Input: dimensioned drawing with shaded views. Units: mm. Origin: part minimum x, y, z. A direction names the side the tool comes from. Give positions to 0.01 mm unless a question says otherwise; leave off trailing zeros. Loops run counter-clockwise (first coordinate to the right, second up) from the corner with the lowest first, then second, coordinate; pieces in that order, holes last. Notation, with made-up numbers: (-32.75, -21) -> (-26.75, -21) arc R24 cw to (-26.75, 2) -> close; hole circle Ø1 at (-14, 72.25). An arc over 180 degrees is marked (long way). One line per question, with ' | ' between items. Start each with the question number.
Item 1: Section A-A on z = 254. Return loops of the section in (x, y) (3 decimals).
Item 2: Section D-D on z = 90. Return loops of the section in (x, y).
Item 3: Set-up query: the marked faces 1, 2, 3, 4 and 5. Return all of +Z, -Z, +X, -X, +Y, -Y with unobstructed straight access to the full face (end or side cutting, diameter ignored); none if empty.
Item 4: Mould query, pull axis Y, two halves, no side actions, for the marked faces 6, 7 and 8. Classes: released by +Y, released by -Y, zero draft, split by the parting line, or undercut.
Item 5: Material intervals for line 1 along X through (y, z) = (37, 254) (3 decimals); line 2 along Z through (x, y) = (500.38, 72.5) (3 decimals); line 3 along X through (y, z) = (296, 251), sorted ascending. Write a range as [from, to].
Item 6: Section C-C on y = 71.5. Return loops of the section in (x, z) (3 decimals), then the cut area to 3 significant figures.
Item 7: Section B-B on x = 500.38. Return loops of the section in (y, z) (3 decimals), then the cut area to 3 significant figures.
Item 8: Pin query (flat end, axial travel): P1, Ø12, axis at x = 339.5, z = 233, coming from the +Y side; P2, Ø12, axis at x = 510.5, z = 182.5, coming from the -Y side. Return the tip coordinate at first contact, or that it passes through.
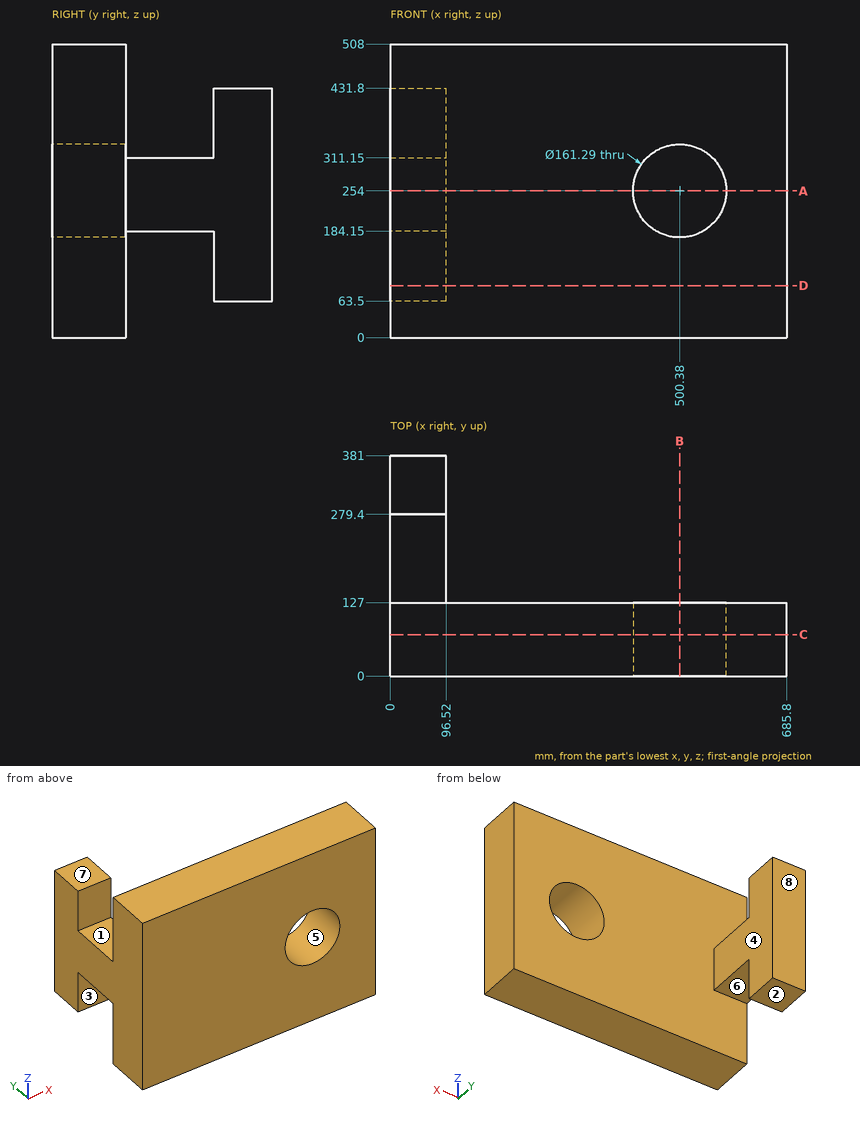
Result sheet:
1) outline: (0, 0) -> (419.735, 0) -> (419.735, 127) -> (96.52, 127) -> (96.52, 381) -> (0, 381) -> close; (581.025, 0) -> (685.8, 0) -> (685.8, 127) -> (581.025, 127) -> close
2) outline: (0, 0) -> (685.8, 0) -> (685.8, 127) -> (0, 127) -> close; (0, 279.4) -> (96.52, 279.4) -> (96.52, 381) -> (0, 381) -> close
3) face 1: +Z, +X, -X | face 2: -Z, +X, -X, +Y | face 3: -Z, +X, -X | face 4: +Z, -Z, +X, +Y | face 5: +Y, -Y
4) face 6: undercut | face 7: zero draft | face 8: released by +Y
5) line 1: x = [0, 419.735], [581.025, 685.8] | line 2: z = [0, 173.355], [334.645, 508] | line 3: x = [0, 96.52]
6) outline: (0, 0) -> (685.8, 0) -> (685.8, 508) -> (0, 508) -> close; hole circle Ø161.29 at (500.38, 254) | area: 328,000 mm²
7) outline: (0, 0) -> (127, 0) -> (127, 173.355) -> (0, 173.355) -> close; (0, 334.645) -> (127, 334.645) -> (127, 508) -> (0, 508) -> close | area: 44,000 mm²
8) P1: stops at y = 127 | P2: passes through
